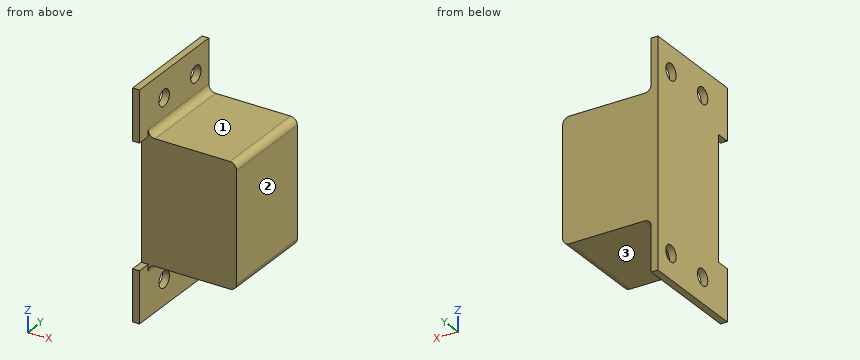
from build123d import *

# Parameters (mm, degrees)
F1_DEPTH = 25.4
F3_D     = 3.7973
F4_W     = 3.175
F4_H     = 28.575
F5_DEPTH = 22.226
F6_R     = 1.5875


with BuildPart() as f1:
    # F0 (on Front) → F1 (new body)
    with BuildSketch(Plane.XZ):
        Polygon((0, 26.19375), (0, 0), (0, -26.19375), (1.5875, -26.19375), (1.5875, -14.2875), (22.225, -14.2875), (22.225, 0), (22.225, 14.2875), (1.5875, 14.2875), (1.5875, 26.19375), align=None)
    extrude(amount=F1_DEPTH)

    # F3 (through all)
    with Locations(Plane.YZ.offset(1.5875)):
        with Locations((-16.35125, 20.32), (-4.7625, 20.32), (-16.35125, -20.32), (-4.7625, -20.32)):
            Hole(F3_D / 2)

    # F4 (on face) → F5 (cut, through all)
    with BuildSketch(Plane.YZ.offset(22.225)):
        with Locations((-23.8125, 0)):
            Rectangle(F4_W, F4_H)
    extrude(amount=-F5_DEPTH, mode=Mode.SUBTRACT)

    # F6
    f6_edges = [f1.edges().sort_by_distance(p)[0] for p in [
        (22.225, -11.1125, 14.2875),
        (22.225, -11.1125, -14.2875),
        (1.5875, -11.1125, 14.2875),
        (1.5875, -11.1125, -14.2875),
    ]]
    fillet(f6_edges, radius=F6_R)


solid = f1.part
The model under review builds one solid part; all positions refer to its coordinate system, in mm. Face numbers are marked on the shaded views. A direction names the side the tool comes from. Give positions to 0.01 mm unless a question says otherwise; leave off trailing zeros. Loops run counter-clockwise (first coordinate to the right, second up) from the corner with the lowest first, then second, coordinate; pieces in that order, holes last. Notation, with made-up numbers: (11.25, 37.5) -> (41.25, 37.5) arc R14 ccw to (41.25, 60.5) -> close; hole circle Ø9 at (3.25, -21). An arc over 180 degrees is marked (long way). Write each question's results on one line, items separated by ' | '.
1) Take a section at B-B, the plane y = -17.5. Give the boundary of the cut face in (x, z) (1 decimal).
Conclusion:
outline: (0, -26.2) -> (1.6, -26.2) -> (1.6, -21.8) -> (0, -21.8) -> close; (0, -18.8) -> (1.6, -18.8) -> (1.6, -15.9) arc R1.6 cw to (3.2, -14.3) -> (20.6, -14.3) arc R1.6 ccw to (22.2, -12.7) -> (22.2, 12.7) arc R1.6 ccw to (20.6, 14.3) -> (3.2, 14.3) arc R1.6 cw to (1.6, 15.9) -> (1.6, 18.8) -> (0, 18.8) -> close; (0, 21.8) -> (1.6, 21.8) -> (1.6, 26.2) -> (0, 26.2) -> close
2) Insertion check: pin 1 Ø9.5 at (y, z) = (-15.5, 22) entering from +X; pin 2 Ø5 at (x, y) = (14.5, -14) entering from -Z; pin 3 Ø11 at (x, z) = (8, 1) entering from -Y (3 decimals); pin 4 Ø2.5 at (y, z) = (-16.35, -20.32) entering from +X. Each pin has a flat end and moves straight along its axis. Give the tip position at first contact, or say it passes through.
Conclusion:
pin 1: stops at x = 1.59 | pin 2: stops at z = -14.29 | pin 3: stops at y = -22.225 | pin 4: passes through
3) Tool access review of the marked faces 1, 2 and 3: name each direction out of +Z, -Z, +X, -X, +Y, -Y from which nothing blocks a thin tool from reaching the whole face with its end or side.
Conclusion:
face 1: +Z, +X, +Y, -Y | face 2: +Z, -Z, +X, +Y, -Y | face 3: -Z, +X, +Y, -Y
4) For line 1 along Z through (x, y) = (13, -8); line 2 along Y through (x, z) = (12.25, -3) (3 decimals); line 3 along X through (y, z) = (-24.5, -21), list the stretches that pass through material, from the lowest coordinate up. Write a range as from..to.
Conclusion:
line 1: z = -14.29..14.29 | line 2: y = -22.225..0 | line 3: x = 0..1.59
5) Take a section at A-A, the plane z = -20.32. Give the boundary of the cut face in (x, y).
Conclusion:
outline: (0, -25.4) -> (1.59, -25.4) -> (1.59, -18.25) -> (0, -18.25) -> close; (0, -14.45) -> (1.59, -14.45) -> (1.59, -6.66) -> (0, -6.66) -> close; (0, -2.86) -> (1.59, -2.86) -> (1.59, 0) -> (0, 0) -> close
6) Take a section at D-D, the plane x = 14. Give the boundary of the cut face in (y, z) (1 decimal), plus the area to 3 significant figures.
Conclusion:
outline: (-22.2, -14.3) -> (0, -14.3) -> (0, 14.3) -> (-22.2, 14.3) -> close | area: 635 mm^2
7) Take a section at C-C, the plane y = -10.75. Give the boundary of the cut face in (x, z) (1 decimal).
Conclusion:
outline: (0, -26.2) -> (1.6, -26.2) -> (1.6, -15.9) arc R1.6 cw to (3.2, -14.3) -> (20.6, -14.3) arc R1.6 ccw to (22.2, -12.7) -> (22.2, 12.7) arc R1.6 ccw to (20.6, 14.3) -> (3.2, 14.3) arc R1.6 cw to (1.6, 15.9) -> (1.6, 26.2) -> (0, 26.2) -> close
